Build history of the part. All positions in model axes, mm. Face numbers are marked on the shaded views. A direction names the side the tool comes from. Round coordinates to 2 decimals unless told otherwise and drop trailing zeros. Write each loop counter-clockwise with the first axis right and the second up, starting at its lowest first coordinate (ties: lowest second). Pieces come first, ordered by that corner, then holes.
1) Which spindle directions (+Z, -Z, +X, -X, +Y, -Y) get a long thin tool onto all of the face, cutting with end or side? Do the marked faces 4, 5 and 6. Say none if no direction does.
2) Saw through at B-B (z = 0). Write the cut outline in (x, y), plus the area to 3 significant figures.
3) Saw through at D-D (x = 2.25). Write the cut outline in (y, z).
4) Wall check: probe 1 along X at (y, z) = (6.15, 0); probe 2 along X at (y, z) = (0.05, 0); probe 3 along Y at (x, z) = (2, -0.5). Give the ranges that are in metal, low to high.
5) Flat gauge pins, fed straight in: pin 1 (3 mm diameter, centred on x = 1, y = 3, fed in from -Z); pin 2 (3 mm diameter, centred on x = -2.5, y = 5, fed in from +Z). Where does each tip first touch, or does it go through?
6) Saw through at A-A (x = 0). Write the cut outline in (y, z).
7) Saw through at C-C (y = 4). Write the cut outline in (x, z).
8) Pull direction Z, two halves, no side cores. Call the marked faces 1, 2 and 3: +Z half, -Z half, draft (parallel to the pull), parting line (faces both ways), or undercut.
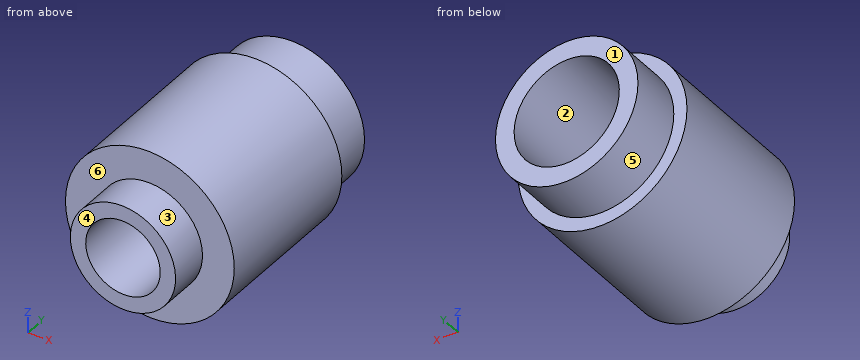
from build123d import *

# Parameters (mm, degrees)
SKETCH1_R           = 3.85
BOSS_EXTRUDE1_DEPTH = 7.2
SKETCH3_R           = 3.25
SKETCH3_R_2         = 2.4
BOSS_EXTRUDE2_DEPTH = 8
SKETCH4_R           = 2.4
CUT_EXTRUDE2_DEPTH  = 5.6
BOSS_EXTRUDE3_START = -5.6
SKETCH5_R           = 2.4
SKETCH5_R_2         = 1.7
BOSS_EXTRUDE3_DEPTH = 5.6
SKETCH6_R           = 1.7
CUT_EXTRUDE3_DEPTH  = 12.036530252


with BuildPart() as part:
    # Sketch1 → Boss-Extrude1 (new body)
    with BuildSketch(Plane(origin=(0, 0, 0), x_dir=(1, 0, 0), z_dir=(0, 1, 0))):
        with Locations(Location((0, 0, 0), (0, 0, 270))):
            Circle(SKETCH1_R)
    extrude(amount=BOSS_EXTRUDE1_DEPTH)

    # Sketch3 → Boss-Extrude2 (add)
    with BuildSketch(Plane(origin=(0, 9.6, 0), x_dir=(1, 0, 0), z_dir=(0, 1, 0))):
        with Locations(Location((0, 0, 0), (0, 0, 270))):
            Circle(SKETCH3_R)
        with Locations(Location((0, 0, 0), (0, 0, 270))):
            Circle(SKETCH3_R_2, mode=Mode.SUBTRACT)
    extrude(amount=-BOSS_EXTRUDE2_DEPTH)

    # Sketch4 → Cut-Extrude2 (cut)
    with BuildSketch(Plane(origin=(0, 7.2, 0), x_dir=(1, 0, 0), z_dir=(0, 1, 0))):
        with Locations(Location((0, 0, 0), (0, 0, 270))):
            Circle(SKETCH4_R)
    extrude(amount=-CUT_EXTRUDE2_DEPTH, mode=Mode.SUBTRACT)

    # Sketch5 → Boss-Extrude3 (add)
    with BuildSketch(Plane(origin=(0, -1.8, 0), x_dir=(-1, 0, 0), z_dir=(0, -1, 0)).offset(BOSS_EXTRUDE3_START)):
        with Locations(Location((0, 0, 0), (0, 0, 270))):
            Circle(SKETCH5_R)
        with Locations(Location((0, 0, 0), (0, 0, 90))):
            Circle(SKETCH5_R_2, mode=Mode.SUBTRACT)
    extrude(amount=BOSS_EXTRUDE3_DEPTH)

    # Sketch6 → Cut-Extrude3 (cut, through all)
    with BuildSketch(Plane.XZ):
        with Locations(Location((0, 0, 0), (0, 0, 270))):
            Circle(SKETCH6_R)
    extrude(amount=-CUT_EXTRUDE3_DEPTH, mode=Mode.SUBTRACT)


solid = part.part
Evaluation:
1. face 4: +Z, -Z, +X, -X, -Y
1. face 5: +Y
1. face 6: -Y
2. outline: (-3.85, 0) - (-2.4, 0) - (-2.4, -1.8) - (-1.7, -1.8) - (-1.7, 3.8) - (-2.4, 3.8) - (-2.4, 9.6) - (-3.25, 9.6) - (-3.25, 7.2) - (-3.85, 7.2) - close; (1.7, -1.8) - (2.4, -1.8) - (2.4, 0) - (3.85, 0) - (3.85, 7.2) - (3.25, 7.2) - (3.25, 9.6) - (2.4, 9.6) - (2.4, 3.8) - (1.7, 3.8) - close
2. area: 32.8 mm2
3. outline: (-1.8, -0.84) - (0, -0.84) - (0, -3.12) - (7.2, -3.12) - (7.2, -2.35) - (9.6, -2.35) - (9.6, -0.84) - (3.8, -0.84) - (3.8, 0.84) - (9.6, 0.84) - (9.6, 2.35) - (7.2, 2.35) - (7.2, 3.12) - (0, 3.12) - (0, 0.84) - (-1.8, 0.84) - close
4. probe 1: x = -3.85 to -2.4, 2.4 to 3.85
4. probe 2: x = -3.85 to -1.7, 1.7 to 3.85
4. probe 3: y = -1.8 to 3.8
5. pin 1: stops at z = -3.85
5. pin 2: stops at z = 3.72
6. outline: (-1.8, -2.4) - (0, -2.4) - (0, -3.85) - (7.2, -3.85) - (7.2, -3.25) - (9.6, -3.25) - (9.6, -2.4) - (3.8, -2.4) - (3.8, -1.7) - (-1.8, -1.7) - close; (-1.8, 1.7) - (3.8, 1.7) - (3.8, 2.4) - (9.6, 2.4) - (9.6, 3.25) - (7.2, 3.25) - (7.2, 3.85) - (0, 3.85) - (0, 2.4) - (-1.8, 2.4) - close
7. outline: circle Ø7.7 at (0, 0); hole circle Ø4.8 at (0, 0)
8. face 1: draft
8. face 2: undercut
8. face 3: parting line
